Part model, mm, in its own coordinate system. A direction names the side the tool comes from. Give positions to 0.01 mm unless a question says otherwise; leave off trailing zeros. Write each loop counter-clockwise with the first axis right and the second up, starting at its lowest first coordinate (ties: lowest second). Pieces come first, ordered by that corner, then holes. Notation, with made-up numbers: M 8.5,-25 L 47.5,-25 A22 cw 47.5,-5 Z; hole C 41.25,83 d8. An arc over 180 degrees is marked long. Answer as CSV lines item,"result". Start each with the question number.
1) Mould opens along Z. For faces 4 (the cylindrical face through (-2.455, -32.715, -36.043)), 5 (the cylindrical face through (8.381, 16.824, 12.8)), 6 (the flat face through (0, -22, -36)) say: pulls with the +Z half, pulls with the -Z half, needs draft (parallel to the pull), parting line crosses it, or undercut.
2) Slice it at D-D, the plane x = 57. Give the cut face in (y, z), plus the area to 3 significant figures.
3) Tool access for faces 1 (the flat face through (29, -27, -31.081)), 2 (the flat face through (-2, -5.098, -36)), 3 (the cylindrical face through (38.58, -33.02, -28.13)): list every direction of +Z, -Z, +X, -X, +Y, -Y with a clear straight run to the whole face (end or side of a thin tool).
4) Slice it at A-A, the plane z = 12. Give the cut face in (x, y).
5) Wall check: line 1 along Z through (x, y) = (15, -12); line 2 along Y through (x, z) = (8, 0); line 3 along Y through (x, z) = (64.5, -27.5). Give the ranges that are in metal, low to high. Write a range as from..to.
6) Pin check, flat tips, straight feed: pin 1 Ø3 at (x, y) = (63.42, -33.1) entering from -Z; pin 2 Ø4.5 at (x, y) = (36.93, -33.1) entering from +Z; pin 3 Ø8 at (x, z) = (62.5, -27) entering from +Y; pin 4 Ø12 at (y, z) = (-23.5, 13) entering from -X. Stop position of each tip, or through.
7) Slice it at C-C, the plane x = 10. Give the cut face in (y, z), plus the area to 3 significant figures.
8) Slice it at B-B, the plane y = 15. Give the cut face in (x, z).
```python
from build123d import *

# Parameters (mm, degrees)
SKETCH1_R                             = 21.14
SKETCH1_R_2                           = 16.14
BOSS_EXTRUDE1_DEPTH                   = 17
BOSS_EXTRUDE2_DEPTH                   = 17
SKETCH3_W                             = 6
SKETCH3_H                             = 34.7
BOSS_EXTRUDE3_DEPTH                   = 60
CUT_EXTRUDE1_DEPTH                    = 30
FILLET1_R                             = 5
BOSS_EXTRUDE4_DEPTH                   = 5
FILLET2_R                             = 5
TAP_DRILL_FOR_M4X0_7_TAP1_D           = 3.3
TAP_DRILL_FOR_M4X0_7_TAP1_DEPTH       = 5
TAP_DRILL_FOR_M4X0_7_TAP1_CSINK_D     = 3.35
TAP_DRILL_FOR_M4X0_7_TAP1_CSINK_ANGLE = 100
TAP_DRILL_FOR_M4X0_7_TAP1_TIP         = 0.991420021
TAP_DRILL_FOR_M4X0_7_TAP2_D           = 3.3
TAP_DRILL_FOR_M4X0_7_TAP2_DEPTH       = 7
TAP_DRILL_FOR_M4X0_7_TAP2_CSINK_D     = 3.35
TAP_DRILL_FOR_M4X0_7_TAP2_CSINK_ANGLE = 100
TAP_DRILL_FOR_M4X0_7_TAP2_TIP         = 0.991420021


with BuildPart() as part:
    # Sketch1 → Boss-Extrude1 (new body)
    with BuildSketch(Plane(origin=(0, 0, 0), x_dir=(0, 0, -1), z_dir=(1, 0, 0))):
        Circle(SKETCH1_R)
        Circle(SKETCH1_R_2, mode=Mode.SUBTRACT)
    extrude(amount=BOSS_EXTRUDE1_DEPTH)

    # Sketch2 → Boss-Extrude2 (add)
    with BuildSketch(Plane.ZY):
        with BuildLine():
            Line((-31.080697416, -39.798400642), (-31.080697416, -5.098400642))
            Line((-31.080697416, -5.098400642), (-16.538596663, 13.167172074))
            ThreePointArc((-16.538596663, 13.167172074), (-13.167172074, -16.538596663), (16.538596663, -13.167172074))
            Line((16.538596663, -13.167172074), (-4.663804983, -39.798400642))
            Line((-4.663804983, -39.798400642), (-31.080697416, -39.798400642))
        make_face()
    extrude(amount=-BOSS_EXTRUDE2_DEPTH)

    # Sketch3 → Boss-Extrude3 (add)
    with BuildSketch(Plane(origin=(17, 0, 0), x_dir=(0, 0, -1), z_dir=(1, 0, 0))):
        with Locations((28.080697416, -22.448400642)):
            Rectangle(SKETCH3_W, SKETCH3_H)
    extrude(amount=BOSS_EXTRUDE3_DEPTH)

    # Sketch4 → Cut-Extrude1 (cut)
    with BuildSketch(Plane.XY.offset(-25.080697416)):
        Polygon((17, -5.098400642), (77, -22.448400642), (77, -5.098400642), align=None)
    extrude(amount=-CUT_EXTRUDE1_DEPTH, mode=Mode.SUBTRACT)

    # Fillet1
    fillet1_edges = [part.edges().sort_by_distance(p)[0] for p in [
        (17, -5.098400642, -28.080697416),
        (17, -22.448400642, -25.080697416),
        (77, -22.448400642, -28.080697416),
    ]]
    fillet(fillet1_edges, radius=FILLET1_R)

    # Sketch5 → Boss-Extrude4 (add)
    with BuildSketch(Plane.ZY):
        Polygon((-31.080697416, -5.098400642), (-41.06651396, -5.098400642), (-41.06651396, -39.798400642), (-25.501919328, -39.798400642), (-4.663804983, -39.798400642), align=None)
    extrude(amount=BOSS_EXTRUDE4_DEPTH)

    # Fillet2
    # the kernel refuses this fillet: 5 mm, written as the material it adds along each edge
    with BuildSketch(Plane(origin=(0, -49.744226019, 2.907889517), x_dir=(0, 0.6057355599289151, 0.795666030089009), z_dir=(0, 0.795666030089009, -0.6057355599289151))) as fillet2_piece_1_section:
        with BuildLine():
            CenterArc((FILLET2_R, -FILLET2_R), FILLET2_R, 90, 90)
            Line((0, -FILLET2_R), (0, 0))
            Line((0, 0), (FILLET2_R, 0))
        make_face()
    fillet2_piece_1 = extrude(amount=68.611262374, mode=Mode.PRIVATE)
    fillet2_piece_1 = split(fillet2_piece_1, bisect_by=Plane(origin=(-1.148121472, -8.497406794, -33.786809657), z_dir=(0, -0.6228558218455279, 0.7823366444141115)), keep=Keep.TOP, mode=Mode.PRIVATE)
    fillet2_piece_1 = split(fillet2_piece_1, bisect_by=Plane(origin=(-1.148121472, -34.831750942, -0.709616331), z_dir=(0, 0.6228558218455282, -0.7823366444141113)), keep=Keep.TOP, mode=Mode.PRIVATE)
    fillet2_piece_1 = split(fillet2_piece_1, bisect_by=Plane(origin=(-1.148121472, -39.798400642, -16.823425528), z_dir=(0, 1, 0)), keep=Keep.TOP, mode=Mode.PRIVATE)
    add(fillet2_piece_1)
    # the kernel refuses this fillet: 5 mm, written as the material it takes off along each edge
    with BuildSketch(Plane(origin=(-5, 7.401599358, -41.06651396), x_dir=(0, 0, 1), z_dir=(0, -1, 0))) as fillet2_2_piece_1:
        with BuildLine():
            CenterArc((FILLET2_R, -FILLET2_R), FILLET2_R, 90, 90)
            Line((0, -FILLET2_R), (0, 0))
            Line((0, 0), (FILLET2_R, 0))
        make_face()
    extrude(amount=59.7, mode=Mode.SUBTRACT)

    # Tap Drill for M4x0.7 Tap1
    with Locations(Plane.ZY.offset(5)):
        with Locations((-35.156261267, -14.70127854), (-35.156261267, -34.106690994)):
            CounterSinkHole(TAP_DRILL_FOR_M4X0_7_TAP1_D / 2, TAP_DRILL_FOR_M4X0_7_TAP1_CSINK_D / 2, depth=TAP_DRILL_FOR_M4X0_7_TAP1_DEPTH, counter_sink_angle=TAP_DRILL_FOR_M4X0_7_TAP1_CSINK_ANGLE)
            with Locations((0, 0, -(TAP_DRILL_FOR_M4X0_7_TAP1_DEPTH + TAP_DRILL_FOR_M4X0_7_TAP1_TIP / 2))):  # 118° drill point
                Cone(0, TAP_DRILL_FOR_M4X0_7_TAP1_D / 2, TAP_DRILL_FOR_M4X0_7_TAP1_TIP, mode=Mode.SUBTRACT)

    # Tap Drill for M4x0.7 Tap2
    with Locations(Plane.XY.offset(-25.080697416)):
        with Locations((36.93257039, -33.095127913), (63.418354043, -33.095127913)):
            CounterSinkHole(TAP_DRILL_FOR_M4X0_7_TAP2_D / 2, TAP_DRILL_FOR_M4X0_7_TAP2_CSINK_D / 2, depth=TAP_DRILL_FOR_M4X0_7_TAP2_DEPTH, counter_sink_angle=TAP_DRILL_FOR_M4X0_7_TAP2_CSINK_ANGLE)
            with Locations((0, 0, -(TAP_DRILL_FOR_M4X0_7_TAP2_DEPTH + TAP_DRILL_FOR_M4X0_7_TAP2_TIP / 2))):  # 118° drill point
                Cone(0, TAP_DRILL_FOR_M4X0_7_TAP2_D / 2, TAP_DRILL_FOR_M4X0_7_TAP2_TIP, mode=Mode.SUBTRACT)


solid = part.part
```
Found:
1,face 4,"undercut"
1,face 5,"parting line crosses it"
1,face 6,"needs draft"
2,outline,"M -39.8,-31.08 L -16.67,-31.08 L -16.67,-25.08 L -39.8,-25.08 Z"
2,area,"139 mm²"
3,face 1,"-Z, +X, +Y, -Y"
3,face 2,"-Z, +X, -X, +Y"
3,face 3,"+Z, -Z"
4,outline,"M 0,-18.87 L 17,-18.87 L 17,-10.79 L 0,-10.79 Z; M 0,10.79 L 17,10.79 L 17,17.4 L 0,17.4 Z"
5,line 1,"-31.08..-10.79, 10.79..17.4"
5,line 2,"-33.94..-16.14, 16.14..21.14"
5,line 3,"-39.8..-34.34, -31.85..-18.83"
6,pin 1,"through"
6,pin 2,"z = -25.08"
6,pin 3,"y = -17.1"
6,pin 4,"x = 0"
7,outline,"M -39.8,-31.08 L -5.1,-31.08 L 13.17,-16.54 A21.14 ccw -13.17,16.54 L -39.8,-4.66 Z; hole C 0,0 d32.28"
7,area,"1,560 mm²"
8,outline,"M 0,-14.9 L 17,-14.9 L 17,-5.96 L 0,-5.96 Z; M 0,5.96 L 17,5.96 L 17,14.9 L 0,14.9 Z"
